from build123d import *

# Parameters (mm, degrees)
BOSS_EXTRUDE1_DEPTH         = 60.96
SKETCH4_R                   = 2.0574
CUT_EXTRUDE3_DEPTH          = 7.35
SKETCH3_R                   = 13.589
SKETCH3_R_2                 = 2.54
CUT_EXTRUDE2_DEPTH          = 13.7
CUT_EXTRUDE4_DEPTH          = 12.7
SKETCH10_W                  = 6.35
SKETCH10_H                  = 25.4
CUT_EXTRUDE5_DEPTH          = 22.86
F_1_4_20_TAPPED_HOLE1_D     = 5.1054
F_1_4_20_TAPPED_HOLE1_DEPTH = 16.51
F_1_4_20_TAPPED_HOLE1_TIP   = 1.533816902


with BuildPart() as part:
    # Sketch1 → Boss-Extrude1 (new body)
    with BuildSketch(Plane(origin=(0, 0, 0), x_dir=(1, 0, 0), z_dir=(0, 1, 0))):
        Polygon((-44.45, 12.7), (-44.45, 0), (0, 0), (0, 38.1), (-6.35, 38.1), (-6.35, 12.7), align=None)
    extrude(amount=BOSS_EXTRUDE1_DEPTH)

    # Sketch4 → Cut-Extrude3 (cut, through all)
    with BuildSketch(Plane.ZY.offset(6.35)):
        with Locations((-25.4, 16.4338)):
            Circle(SKETCH4_R)
        with Locations((-25.4, 27.686)):
            Circle(SKETCH4_R)
    extrude(amount=-CUT_EXTRUDE3_DEPTH, mode=Mode.SUBTRACT)

    # Sketch3 → Cut-Extrude2 (cut, through all)
    with BuildSketch(Plane(origin=(0, 0, -12.7), x_dir=(-1, 0, 0), z_dir=(0, 0, -1))):
        with Locations((19.939, 39.9796)):
            Circle(SKETCH3_R)
        with Locations((35.179, 55.2196)):
            Circle(SKETCH3_R_2)
        with Locations((11.049, 55.2196)):
            Circle(SKETCH3_R_2)
        with Locations((11.049, 24.7396)):
            Circle(SKETCH3_R_2)
        with Locations((35.179, 24.7396)):
            Circle(SKETCH3_R_2)
    extrude(amount=-CUT_EXTRUDE2_DEPTH, mode=Mode.SUBTRACT)

    # Sketch6 → Cut-Extrude4 (cut)
    with BuildSketch(Plane.XZ):
        Polygon((-47.891108231, 6.866314065), (10.481478335, -42.114101793), (8.522261701, -44.449005256), (-49.850324865, 4.531410602), align=None)
    extrude(amount=-CUT_EXTRUDE4_DEPTH, mode=Mode.SUBTRACT)

    # Sketch10 → Cut-Extrude5 (cut)
    with BuildSketch(Plane(origin=(0, 60.96, 0), x_dir=(1, 0, 0), z_dir=(0, 1, 0))):
        with Locations((-3.175, 25.4)):
            Rectangle(SKETCH10_W, SKETCH10_H)
    extrude(amount=-CUT_EXTRUDE5_DEPTH, mode=Mode.SUBTRACT)

    # 1/4-20 Tapped Hole1
    with Locations(Plane.XY):
        with Locations((-35.179, 55.2196), (-11.049, 55.2196), (-35.179, 24.7396), (-11.049, 24.7396)):
            Hole(F_1_4_20_TAPPED_HOLE1_D / 2, depth=F_1_4_20_TAPPED_HOLE1_DEPTH)
            with Locations((0, 0, -(F_1_4_20_TAPPED_HOLE1_DEPTH + F_1_4_20_TAPPED_HOLE1_TIP / 2))):  # 118° drill point
                Cone(0, F_1_4_20_TAPPED_HOLE1_D / 2, F_1_4_20_TAPPED_HOLE1_TIP, mode=Mode.SUBTRACT)


solid = part.part
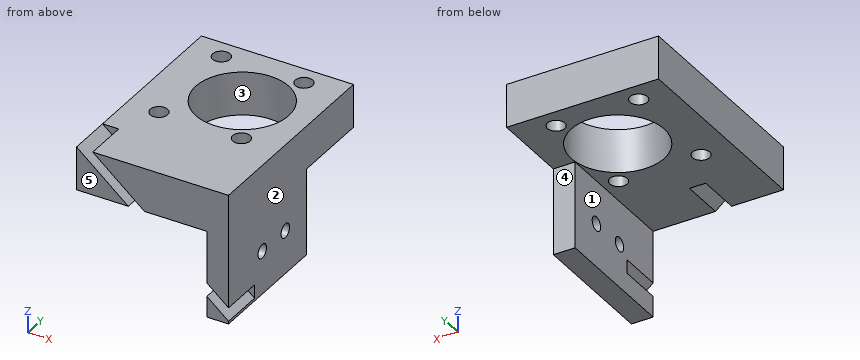
Model file for the job. Use its own axes, mm. Face numbers are marked on the shaded views. A direction names the side the tool comes from. Give positions to 0.01 mm unless a question says otherwise; leave off trailing zeros. Loops run counter-clockwise (first coordinate to the right, second up) from the corner with the lowest first, then second, coordinate; pieces in that order, holes last.
Item 1: Mould opens along X. For the marked faces 1, 2 and 3 say: +X half, -X half, draft (parallel to the pull), parting line (faces both ways), or undercut.
Check values:
face 1: -X half
face 2: +X half
face 3: undercut
Item 2: Slice it at D-D (x = -28.5). Write the cut outline in (y, z), plus the area to 3 significant figures.
Check values:
outline: (0, -9.4) - (12.7, -9.4) - (12.7, -12.7) - (29.43, -12.7) - (29.43, 0) - (0, 0) - close; (50.53, -12.7) - (60.96, -12.7) - (60.96, 0) - (50.53, 0) - close
area: 464 mm2
Item 3: Slice it at B-B (z = -25.4). Write the cut outline in (x, y).
Check values:
outline: (-6.35, 0) - (0, 0) - (0, 14.38) - (-6.35, 14.38) - close; (-6.35, 18.49) - (0, 18.49) - (0, 25.63) - (-6.35, 25.63) - close; (-6.35, 29.74) - (0, 29.74) - (0, 38.1) - (-6.35, 38.1) - close
Item 4: Slice it at A-A (y = 11). Write the cut outline in (x, z).
Check values:
outline: (-44.45, -12.7) - (-29.31, -12.7) - (-44.45, 0) - close; (-39.71, 0) - (-24.57, -12.7) - (-6.35, -12.7) - (-6.35, -27.99) - (0, -33.32) - (0, 0) - close; (-6.35, -38.1) - (0, -38.1) - (0, -37.3) - (-6.35, -31.97) - close
Item 5: Drop flat-ended pins along their axis: P1, Ø4.5, axis at y = 27.686, z = -25.4, coming from the -X side; P2, Ø21.5, axis at x = -19.94, y = 39.98, coming from the +Z side; P3, Ø6, axis at x = -35.18, y = 55.22, coming from the -Z side; P4, Ø3, axis at x = -3.5, z = -29, coming from the +Y side. Give the stop position or say it passes through.
Check values:
P1: stops at x = -6.35
P2: passes through
P3: stops at z = -12.7
P4: stops at y = 38.1
Item 6: Which spindle directions (+Z, -Z, +X, -X, +Y, -Y) get a long thin tool onto all of the face, cutting with end or side? Do the marked faces 4 and 5. Say none if no direction does.
Check values:
face 4: -Z, +X, -X, +Y
face 5: +Z, -Z, +X, -X, -Y
Item 7: Drill centre lines: line 1 along Y through (x, z) = (-1.75, -25.4); line 2 along Y through (x, z) = (-1, -25); line 3 along X through (y, z) = (24, -4.5). Where is each one in solid material? Low to high.
Check values:
line 1: y = 0 to 14.38, 18.49 to 25.63, 29.74 to 38.1
line 2: y = 0 to 14.42, 18.45 to 25.67, 29.7 to 38.1
line 3: x = -44.45 to -37.62, -32.74 to -13.49, -8.61 to 0
Item 8: Slice it at C-C (x = -36). Write the cut outline in (y, z), plus the area to 3 significant figures.
Check values:
outline: (0, -12.7) - (22.32, -12.7) - (22.32, 0) - (0, 0) - (0, -3.11) - (12.7, -3.11) - (12.7, -7.09) - (0, -7.09) - close; (27.16, -12.7) - (52.8, -12.7) - (52.8, 0) - (27.16, 0) - close; (57.64, -12.7) - (60.96, -12.7) - (60.96, 0) - (57.64, 0) - close
area: 601 mm2
